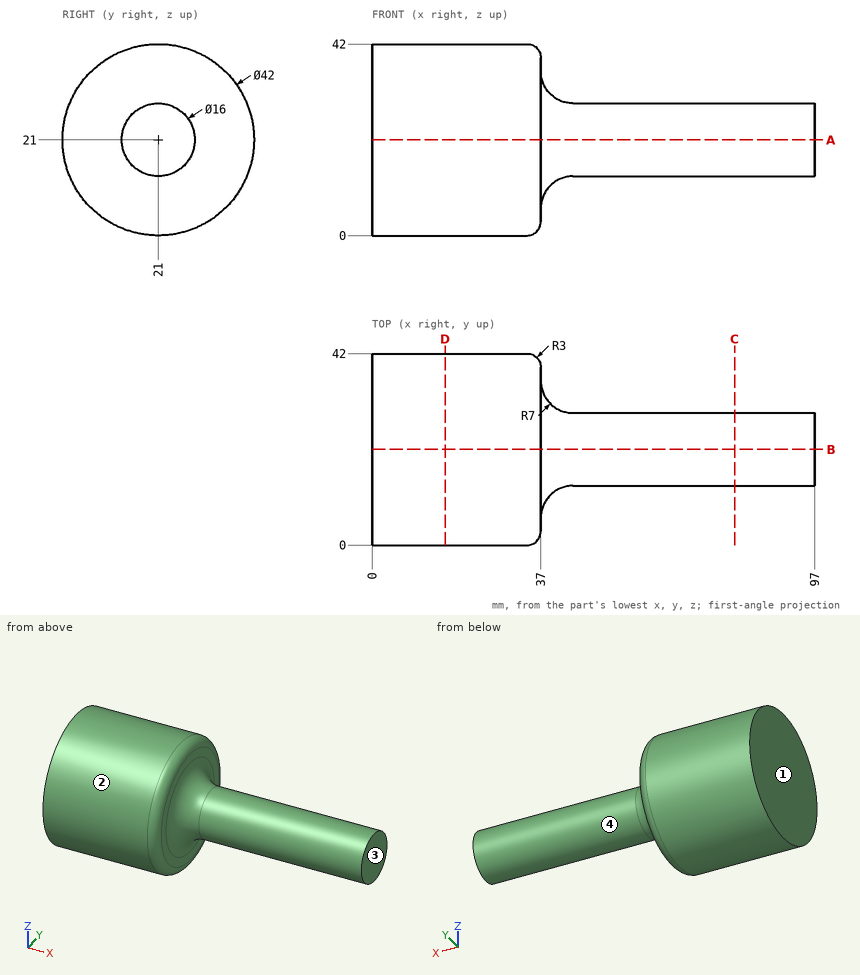
Answer from the drawing. Dimensions are ordinates in mm from the lowest x, y and z of the part. A direction names the side the tool comes from. Round coordinates to 2 decimals unless told otherwise and drop trailing zeros. Write each loop counter-clockwise with the first axis right and the second up, starting at its lowest first coordinate (ties: lowest second). Pieces come first, ordered by that corner, then holes.
1. The part is cut by section C-C, the plane x = 79.5. Determine the outline of the cut face in (y, z).
2. Determine the mould class of the marked faces 1 and 2 for opening direction Z: pulls with the +Z half, pulls with the -Z half, needs draft (parallel to the pull), parting line crosses it, or undercut.
3. Which of the six approach directions +Z, -Z, +X, -X, +Y, -Y give full straight-line access (tool end or side, diameter ignored) to the marked faces 3 and 4?
4. The part is cut by section D-D, the plane x = 16. Determine the outline of the cut face in (y, z).
5. Given pin 1 Ø4 at (x, y) = (75.5, 13.5) entering from +Z; pin 2 Ø12 at (x, z) = (38.5, 8.5) entering from +Y; pin 3 Ø8 at (x, z) = (21.5, 12) entering from -Y, each flat-ended and moving along its own axis, determine where each tip first touches the part or whether it passes through.
6. Straight lines are drawn through the part: L1, parallel to Y at x = 84, z = 21.5; L2, parallel to X at y = 14, z = 37; L3, parallel to X at y = 9.5, z = 5. For each, find the intervals that lie inside material, in ascending order.
7. The part is cut by section A-A, the plane z = 21. Determine the outline of the cut face in (x, y), then the cut area to 3 significant figures.
Values:
1. outline: circle Ø16 at (21, 21)
2. face 1: needs draft
2. face 2: parting line crosses it
3. face 3: +Z, -Z, +X, +Y, -Y
3. face 4: +X
4. outline: circle Ø42 at (21, 21)
5. pin 1: stops at z = 26.81
5. pin 2: stops at y = 40.39
5. pin 3: stops at y = 0.6
6. L1: y = 13.02 to 28.98
6. L2: x = 0 to 37
6. L3: x = 0 to 36.47
7. outline: (0, 0) - (34, 0) arc R3 ccw to (37, 3) - (37, 6) arc R7 cw to (44, 13) - (97, 13) - (97, 29) - (44, 29) arc R7 cw to (37, 36) - (37, 39) arc R3 ccw to (34, 42) - (0, 42) - close
7. area: 2,530 mm2
